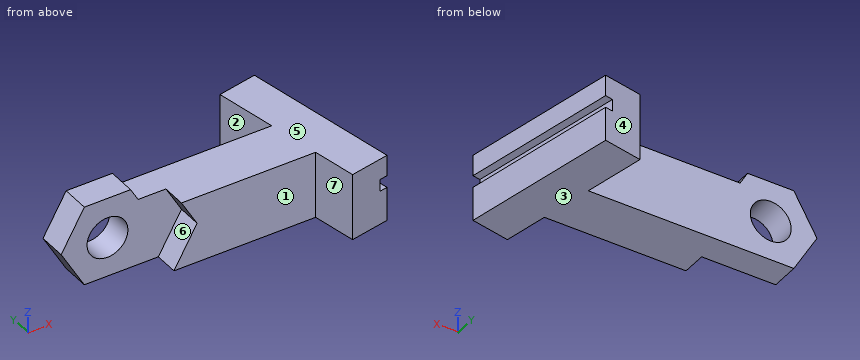
```python
from build123d import *

# Parameters (mm, degrees)
SKETCH1_W                = 25
SKETCH1_H                = 6.75
BOSS_EXTRUDE1_DEPTH      = 6.5
BOSS_EXTRUDE3_DEPTH      = 3.375
BOSS_EXTRUDE3_DEPTH_BACK = 5
SKETCH4_W                = 1
SKETCH4_H                = 1.5
CUT_EXTRUDE1_DEPTH       = 23
BOSS_EXTRUDE4_DEPTH      = 6.5
SKETCH6_R                = 2.55
CUT_EXTRUDE2_DEPTH       = 10
BOSS_EXTRUDE5_REACH      = 12
CUT_EXTRUDE3_DEPTH       = 3


with BuildPart() as part:
    # Sketch1 → Boss-Extrude1 (new body)
    with BuildSketch(Plane(origin=(0, 0, 0), x_dir=(1, 0, 0), z_dir=(0, 1, 0))):
        with Locations((12.5, -3.375)):
            Rectangle(SKETCH1_W, SKETCH1_H)
    extrude(amount=BOSS_EXTRUDE1_DEPTH)

    # Sketch3 → Boss-Extrude3 (add, two sides)
    with BuildSketch(Plane.XY.offset(3.375)) as boss_extrude3_sk:
        Polygon((21.275684175, 14.155521181), (26.183820092, 15.109566157), (30, -4.522977512), (25.091864083, -5.477022488), align=None)
    extrude(amount=BOSS_EXTRUDE3_DEPTH)
    extrude(boss_extrude3_sk.sketch, amount=-BOSS_EXTRUDE3_DEPTH_BACK)

    # Sketch4 → Cut-Extrude1 (cut)
    with BuildSketch(Plane(origin=(-1.876769127, 9.65514015, 0), x_dir=(0.981627183, 0.190808995, 0), z_dir=(-0.190808995, 0.981627183, 0))):
        with Locations((28.085790708, -3.375)):
            Rectangle(SKETCH4_W, SKETCH4_H)
    extrude(amount=-CUT_EXTRUDE1_DEPTH, mode=Mode.SUBTRACT)

    # Sketch5 → Boss-Extrude4 (add)
    with BuildSketch(Plane(origin=(0, 6.5, 0), x_dir=(1, 0, 0), z_dir=(0, 1, 0))):
        Polygon((-5.773502692, -3.375), (-2.886751346, -8.375), (2.886751346, -8.375), (5.773502692, -3.375), (2.886751346, 1.625), (-2.886751346, 1.625), align=None)
    extrude(amount=-BOSS_EXTRUDE4_DEPTH)

    # Sketch6 → Cut-Extrude2 (cut)
    with BuildSketch(Plane(origin=(0, 6.5, 0), x_dir=(1, 0, 0), z_dir=(0, 1, 0))):
        with Locations((0, -3.335615973)):
            Circle(SKETCH6_R)
    extrude(amount=-CUT_EXTRUDE2_DEPTH, mode=Mode.SUBTRACT)

    # Sketch7 → Boss-Extrude5 (add, up to next)
    with BuildSketch(Plane(origin=(0, 0, -1.625), x_dir=(-1, 0, 0), z_dir=(0, 0, -1)), mode=Mode.PRIVATE) as boss_extrude5_sk1:
        Polygon((-2.886751346, 0), (-24.027238758, 0), (-25.091864083, -5.477022488), (-30, -4.522977512), (-26.183820092, 15.109566157), (-21.275684175, 14.155521181), (-22.763766749, 6.5), (-2.886751346, 6.5), align=None)
    boss_extrude5_tool1 = extrude(boss_extrude5_sk1.sketch, amount=-BOSS_EXTRUDE5_REACH, mode=Mode.PRIVATE) - part.part
    add(boss_extrude5_tool1.solids().sort_by_distance((18.499322, 3.902268, -1.625))[0])

    # Sketch8 → Cut-Extrude3 (cut)
    with BuildSketch(Plane(origin=(0, 0, 0), x_dir=(-1, 0, 0), z_dir=(0, -1, 0))):
        Polygon((-4.618802154, -11.375), (4.618802154, -11.375), (9.237604307, -3.375), (4.618802154, 4.625), (-4.618802154, 4.625), (-9.237604307, -3.375), align=None)
    extrude(amount=-CUT_EXTRUDE3_DEPTH, mode=Mode.SUBTRACT)


solid = part.part
```
Geometry check sheet. Reference: the model listing, model coordinates, mm. Face numbers are marked on the shaded views. A direction names the side the tool comes from. Coordinates: 2 decimals unless noted, no trailing zeros. Write each loop counter-clockwise with the first axis right and the second up, starting at its lowest first coordinate (ties: lowest second). Pieces come first, ordered by that corner, then holes. Notation, with made-up numbers: M 8.5,23 L 49.5,23 A16 cw 49.5,33 Z; hole C -34,15.5 d1. An arc over 180 degrees is marked long. Answer as a JSON object with one key per item and string values.
1. Tool access check on the marked faces 5, 6 and 7. Record the directions out of +Z, -Z, +X, -X, +Y, -Y that give a thin tool (end or side, any length) a straight path to the whole face; none if there is none.
Answers below:
{"face 5": "+Z, +X, +Y, -Y", "face 6": "-X, -Y", "face 7": "+Z, -Z, -X, -Y"}
2. Go/stop test with flat-tipped pins: pin 1 Ø2.5 at (x, z) = (13.5, 1) entering from -Y; pin 2 Ø1.5 at (y, z) = (1.5, -0.5) entering from -X; pin 3 Ø2.5 at (x, y) = (26.5, 6) entering from +Z. Record where each tip stops, or that it passes through.
Answers below:
{"pin 1": "stops at y = 0", "pin 2": "stops at x = 6.57", "pin 3": "stops at z = 6.75"}
3. Section check B-B, the plane z = 4.5. Enter the section's corners in (x, y).
Answers below:
{"outline": "M -5.12,3 L -2.27,3 L -2.27,6.5 L -5.12,6.5 Z; M 2.27,3 L 8.59,3 L 8.59,0 L 24.03,0 L 25.09,-5.48 L 30,-4.52 L 26.18,15.11 L 21.28,14.16 L 22.76,6.5 L 2.27,6.5 Z"}
4. Scan lines: L1, parallel to Z at x = 0, y = 4.45 (3 decimals); L2, parallel to Y at x = -3, z = 4.5; L3, parallel to Z at x = 26.5, y = 4.25 (3 decimals). Record each from-to range of solid material in increasing order.
Answers below:
{"L1": "z = -1.625 to 0.786, 5.886 to 8.375", "L2": "y = 3 to 6.5", "L3": "z = -1.625 to 6.75"}
5. Section check D-D, the plane x = 4.5. Enter the section's corners in (y, z) (3 decimals).
Answers below:
{"outline": "M 3,-1.625 L 6.5,-1.625 L 6.5,6.75 L 3,6.75 Z"}
6. Section check A-A, the plane x = 0. Enter the section's corners in (y, z) (3 decimals).
Answers below:
{"outline": "M 3,-1.625 L 6.5,-1.625 L 6.5,0.786 L 3,0.786 Z; M 3,5.886 L 6.5,5.886 L 6.5,8.375 L 3,8.375 Z"}
7. Draft check along Y on the marked faces 1, 2, 3 and 4. Enter one of: released by +Y, released by -Y, zero draft, split by the parting line, or undercut.
Answers below:
{"face 1": "released by -Y", "face 2": "undercut", "face 3": "zero draft", "face 4": "released by +Y"}
